from build123d import *

# Parameters (mm, degrees)
SKETCH1_R           = 1.7526
SKETCH1_W           = 12.7
SKETCH1_H           = 5.742
BOSS_EXTRUDE1_DEPTH = 5.842
SKETCH2_R           = 3.175
CUT_EXTRUDE1_DEPTH  = 82.290714919
FILLET1_R           = 6.35
CUT_EXTRUDE2_DEPTH  = 82.290714919
FILLET2_R           = 1
FILLET3_R           = 3.175
CUT_EXTRUDE3_DEPTH  = 82.290714919


with BuildPart() as part:
    # Sketch1 → Boss-Extrude1 (new body)
    with BuildSketch(Plane.XY):
        with BuildLine():
            Line((-61.722, 0), (-61.722, 12.7))
            Line((-61.722, 12.7), (-55.88, 12.7))
            Line((-55.88, 12.7), (-55.88, 25.4))
            Line((-55.88, 25.4), (-61.722, 25.4))
            Line((-61.722, 25.4), (-61.722, 38.1))
            Line((-61.722, 38.1), (-55.88, 38.1))
            Line((-55.88, 38.1), (-55.88, 44.45))
            Line((-55.88, 44.45), (55.88, 44.45))
            Line((55.88, 44.45), (55.88, -44.45))
            Line((55.88, -44.45), (7.127875, -44.45))
            Line((7.127875, -44.45), (2.573780292, -50.179278348))
            ThreePointArc((2.573780292, -50.179278348), (-2.397125, -52.578), (-7.368030292, -50.179278348))
            Line((-7.368030292, -50.179278348), (-11.922125, -44.45))
            Line((-11.922125, -44.45), (-55.88, -44.45))
            Line((-55.88, -44.45), (-55.88, -37.692))
            Line((-55.88, -37.692), (-29.083, -37.692))
            Line((-29.083, -37.692), (-29.083, -31.85))
            Line((-29.083, -31.85), (-55.88, -31.85))
            Line((-55.88, -31.85), (-55.88, -25.4))
            Line((-55.88, -25.4), (-61.722, -25.4))
            Line((-61.722, -25.4), (-61.722, -12.7))
            Line((-61.722, -12.7), (-55.88, -12.7))
            Line((-55.88, -12.7), (-55.88, -6.25))
            Line((-55.88, -6.25), (-29.083, -6.25))
            Line((-29.083, -6.25), (-29.083, -0.408))
            Line((-29.083, -0.408), (-55.88, -0.408))
            Line((-55.88, -0.408), (-55.88, 0))
            Line((-55.88, 0), (-61.722, 0))
        make_face()
        with Locations((-22.733, -3.329)):
            Circle(SKETCH1_R, mode=Mode.SUBTRACT)
        with Locations((15.367, -3.329)):
            Circle(SKETCH1_R, mode=Mode.SUBTRACT)
        with Locations(Location((15.367, -34.771, 0), (0, 0, 180))):
            Circle(SKETCH1_R, mode=Mode.SUBTRACT)
        with Locations(Location((-22.733, -34.771, 0), (0, 0, 180))):
            Circle(SKETCH1_R, mode=Mode.SUBTRACT)
        with Locations((-5.08, 31.75)):
            Circle(SKETCH1_R, mode=Mode.SUBTRACT)
        with Locations((20.32, 31.75)):
            Circle(SKETCH1_R, mode=Mode.SUBTRACT)
        Polygon((9.017, -0.408), (-10.541, -0.408), (-16.383, -0.408), (-16.383, -6.25), (-10.541, -6.25), (9.017, -6.25), align=None, mode=Mode.SUBTRACT)
        Polygon((27.559, -0.408), (21.717, -0.408), (21.717, -6.25), (27.559, -6.25), (40.259, -6.25), (40.259, -0.408), align=None, mode=Mode.SUBTRACT)
        Polygon((21.717, -37.692), (21.717, -31.85), (27.559, -31.85), (40.259, -31.85), (40.259, -37.692), (27.559, -37.692), align=None, mode=Mode.SUBTRACT)
        Polygon((-16.383, -37.692), (-16.383, -31.85), (-10.541, -31.85), (9.017, -31.85), (9.017, -37.692), (-10.541, -37.692), align=None, mode=Mode.SUBTRACT)
        with BuildLine():
            Line((-2.794, -44.1452), (-2.00025, -44.1452))
            ThreePointArc((-2.00025, -44.1452), (0.08255, -46.228), (-2.00025, -48.3108))
            Line((-2.00025, -48.3108), (-2.794, -48.3108))
            ThreePointArc((-2.794, -48.3108), (-4.8768, -46.228), (-2.794, -44.1452))
        make_face(mode=Mode.SUBTRACT)
        with BuildLine():
            Line((-2.794, 17.5768), (-2.00025, 17.5768))
            ThreePointArc((-2.00025, 17.5768), (0.08255, 15.494), (-2.00025, 13.4112))
            Line((-2.00025, 13.4112), (-2.794, 13.4112))
            ThreePointArc((-2.794, 13.4112), (-4.8768, 15.494), (-2.794, 17.5768))
        make_face(mode=Mode.SUBTRACT)
        with Locations((-17.78, 31.75)):
            Rectangle(SKETCH1_W, SKETCH1_H, mode=Mode.SUBTRACT)
        with Locations((-43.18, 31.75)):
            Rectangle(SKETCH1_W, SKETCH1_H, mode=Mode.SUBTRACT)
        with Locations((7.62, 31.75)):
            Rectangle(SKETCH1_W, SKETCH1_H, mode=Mode.SUBTRACT)
        with Locations((33.02, 31.75)):
            Rectangle(SKETCH1_W, SKETCH1_H, mode=Mode.SUBTRACT)
    extrude(amount=BOSS_EXTRUDE1_DEPTH)

    # Sketch2 → Cut-Extrude1 (cut, through all)
    with BuildSketch(Plane.XY.offset(5.842)):
        with Locations((-51.1175, 15.494)):
            Circle(SKETCH2_R)
    extrude(amount=-CUT_EXTRUDE1_DEPTH, mode=Mode.SUBTRACT)

    # Fillet1
    fillet1_edges = [part.edges().sort_by_distance(p)[0] for p in [
        (7.127875, -44.45, 2.921),
        (-11.922125, -44.45, 2.921),
    ]]
    fillet(fillet1_edges, radius=FILLET1_R)

    # Sketch4 → Cut-Extrude2 (cut, through all)
    with BuildSketch(Plane.XY.offset(5.842)):
        with BuildLine():
            Line((-43.18, 50.8), (-30.48, 50.8))
            ThreePointArc((-30.48, 50.8), (-24.13, 44.45), (-30.48, 38.1))
            Line((-30.48, 38.1), (-43.18, 38.1))
            ThreePointArc((-43.18, 38.1), (-49.53, 44.45), (-43.18, 50.8))
        make_face()
    extrude(amount=-CUT_EXTRUDE2_DEPTH, mode=Mode.SUBTRACT)

    # Fillet2
    fillet2_edges = [part.edges().sort_by_distance(p)[0] for p in [
        (-24.13, 44.45, 2.921),
        (-49.53, 44.45, 2.921),
    ]]
    fillet(fillet2_edges, radius=FILLET2_R)

    # Fillet3
    fillet3_edges = [part.edges().sort_by_distance(p)[0] for p in [
        (55.88, -44.45, 2.921),
    ]]
    fillet(fillet3_edges, radius=FILLET3_R)

    # Sketch5 → Cut-Extrude3 (cut, through all)
    with BuildSketch(Plane.XY.offset(5.842)):
        with BuildLine():
            Line((3.4925, -23.8125), (3.4925, -14.2875))
            ThreePointArc((3.4925, -14.2875), (8.255, -9.525), (13.0175, -14.2875))
            Line((13.0175, -14.2875), (13.0175, -23.8125))
            ThreePointArc((13.0175, -23.8125), (8.255, -28.575), (3.4925, -23.8125))
        make_face()
        with BuildLine():
            Line((3.4925, 17.1545), (3.4925, 7.6295))
            ThreePointArc((3.4925, 7.6295), (8.255, 2.867), (13.0175, 7.6295))
            Line((13.0175, 7.6295), (13.0175, 17.1545))
            ThreePointArc((13.0175, 17.1545), (8.255, 21.917), (3.4925, 17.1545))
        make_face()
    extrude(amount=-CUT_EXTRUDE3_DEPTH, mode=Mode.SUBTRACT)


solid = part.part
Can you work these out from the model? Positions are in its coordinate system, mm. A direction names the side the tool comes from. Give positions to 0.01 mm unless a question says otherwise; leave off trailing zeros. Order: outer loops, then holes, each group sorted by start corner. A loop starts at its lowest first (then second) coordinate and runs counter-clockwise, first axis right, second up. Notation, with made-up numbers: M 27,-38.75 L 71,-38.75 A21 cw 71,-10.75 Z; hole C 67.25,31.5 d5. An arc over 180 degrees is marked long. One line per item, written item: value.
Item 1: If we section it at A-A on y = -21: Write out the boundary of the cut face in (x, z), and give its area (3 significant figures).
Verdict:
outline: M -61.72,0 L 3.49,0 L 3.49,5.84 L -61.72,5.84 Z; M 13.02,0 L 55.88,0 L 55.88,5.84 L 13.02,5.84 Z
area: 631 mm2
Item 2: If we mould it in two halves opening along Y, with no side actions, what happens to faces 1 (the face through (7.468, -45.064, 2.962)), 2 (the face through (-55.88, -10, 3)), 3 (the face through (33, 34.621, 3)), 4 (the face through (-2, 7, 0))? For each: pulls with the +Y half, pulls with the -Y half, needs draft (parallel to the pull), parting line crosses it, or undercut.
Verdict:
face 1: pulls with the -Y half
face 2: undercut
face 3: undercut
face 4: needs draft
Item 3: Please list where these lines run through material, in increasing order: line 1 (X direction, y = -1.5, z = 5.35); line 2 (Y direction, x = 40, z = 2.2); line 3 (Y direction, x = 37.5, z = 0.6).
Verdict:
line 1: -29.08 to -16.38, 9.02 to 21.72, 40.26 to 55.88
line 2: -44.45 to -37.69, -31.85 to -6.25, -0.41 to 44.45
line 3: -44.45 to -37.69, -31.85 to -6.25, -0.41 to 28.88, 34.62 to 44.45
Item 4: If we section it at B-B on x = 35.5: Write out the boundary of the cut face in (y, z), and give its area (3 significant figures).
Verdict:
outline: M -44.45,0 L -37.69,0 L -37.69,5.84 L -44.45,5.84 Z; M -31.85,0 L -6.25,0 L -6.25,5.84 L -31.85,5.84 Z; M -0.41,0 L 28.88,0 L 28.88,5.84 L -0.41,5.84 Z; M 34.62,0 L 44.45,0 L 44.45,5.84 L 34.62,5.84 Z
area: 418 mm2
Item 5: For pin 1 (3 mm diameter, centred on x = -18, z = 3, fed in from -Y); pin 2 (4 mm diameter, centred on x = -51.12, y = 15.49, fed in from +Z) (1 decimal); pin 3 (3 mm diameter, centred on y = 17, z = 4, fed in from -X); pin 4 (1.8 mm diameter, centred on x = -59.5, z = 4, fed in from +Y), each with a flat end and sliding along its axis, tell me the tip position at first contact or that it passes through.
Verdict:
pin 1: y = -44.45
pin 2: through
pin 3: x = -55.88
pin 4: y = 38.1
Item 6: If we section it at D-D on x = 20.32: Write out the boundary of the cut face in (y, z), and give its area (3 significant figures).
Verdict:
outline: M -44.45,0 L 30,0 L 30,5.84 L -44.45,5.84 Z; M 33.5,0 L 44.45,0 L 44.45,5.84 L 33.5,5.84 Z
area: 499 mm2
Item 7: If we section it at C-C on y = 31.75: Write out the boundary of the cut face in (x, z).
Verdict:
outline: M -61.72,0 L -49.53,0 L -49.53,5.84 L -61.72,5.84 Z; M -36.83,0 L -24.13,0 L -24.13,5.84 L -36.83,5.84 Z; M -11.43,0 L -6.83,0 L -6.83,5.84 L -11.43,5.84 Z; M -3.33,0 L 1.27,0 L 1.27,5.84 L -3.33,5.84 Z; M 13.97,0 L 18.57,0 L 18.57,5.84 L 13.97,5.84 Z; M 22.07,0 L 26.67,0 L 26.67,5.84 L 22.07,5.84 Z; M 39.37,0 L 55.88,0 L 55.88,5.84 L 39.37,5.84 Z
Item 8: For faces 5 (the face through (-59, -25.4, 3)), 6 (the face through (-2, 7, 5.842)), 7 (the face through (32, -44.45, 3)), 8 (the face through (-36.83, 32, 3)), which set-ups out of +Z, -Z, +X, -X, +Y, -Y let a thin tool reach every point of the face, with its end or its side?
Verdict:
face 5: +Z, -Z, -X, -Y
face 6: +Z, +X, -X, +Y, -Y
face 7: +Z, -Z, +X, -Y
face 8: +Z, -Z
